Autodesk Inventor part; units mm, degrees
ref_plane "YZ Plane" through (0, 0, 0) normal (1, 0, 0) x (0, 1, 0)
ref_plane "XZ Plane" through (0, 0, 0) normal (0, 1, 0) x (-1, 0, 0)
ref_plane "XY Plane" through (0, 0, 0) normal (0, 0, 1) x (1, 0, 0)
sketch "Sketch1" plane through (0, 0, 0) normal (0, 0, 1) x (1, 0, 0)
  circle A0 centre (0, 0) radius 82.55
  circle A1 centre (0, 0) radius 101.6
  dimension "d0" = 203.2
  dimension "d1" = 19.05
extrude "Extrusion1" add sketch "Sketch1" along normal blind 4.7625
sketch "Sketch2" plane through (0, 0, 4.7625) normal (0, 0, 1) x (1, 0, 0)
  circle A0 centre (0, 0) radius 101.6
  line L0 (0, 0) -> (0, 92.075) construction
  circle A1 centre (0, 0) radius 92.075 construction
  circle A2 centre (0, 92.075) radius 3.175
  dimension "d4" = 9.525
  dimension "d5" = 6.35
extrude "Extrusion2" cut sketch "Sketch2" against normal through all contours A2
pattern_circular "Circular Pattern1" count 24 over 360 about axis through (0, 0, -10) along (0, 0, 1) of "Extrusion2"
properties part number "FlyWheelWeight" material "Aluminum-6061"
Can you work these out from the model? Positions are in its coordinate system, mm. Coordinates: 2 decimals unless noted, no trailing zeros. Write each loop counter-clockwise with the first axis right and the second up, starting at its lowest first coordinate (ties: lowest second). Pieces come first, ordered by that corner, then holes. Notation, with made-up numbers: M -24.75,-14.75 L 9.25,-14.75 A23 ccw 9.25,10.25 Z; hole C 12,-34.75 d8. An arc over 180 degrees is marked long. Answer as CSV lines item,"result".
Item 1: Imagine slicing it at A-A on y = 0. List the corners of the cut face in (x, z) for me, plus the area to 3 significant figures.
Geometry results:
outline,"M -101.6,0 L -95.25,0 L -95.25,4.76 L -101.6,4.76 Z; M -88.9,0 L -82.55,0 L -82.55,4.76 L -88.9,4.76 Z; M 82.55,0 L 88.9,0 L 88.9,4.76 L 82.55,4.76 Z; M 95.25,0 L 101.6,0 L 101.6,4.76 L 95.25,4.76 Z"
area,"121 mm2"
Item 2: Imagine slicing it at D-D on z = 2.2. State how many separate pieces and enclosed holes the cut face has, plus the area to 3 significant figures.
Geometry results:
separate pieces,"1"
enclosed holes,"25"
area,"10,300 mm2"
Item 3: Please list where these lines run through material, in increasing order: line 1 along Y through (x, z) = (0, 3.65); line 2 along X through (y, z) = (-68, 1.05); line 3 along Y through (x, z) = (65.5, 4.5).
Geometry results:
line 1,"y = -101.6 to -95.25, -88.9 to -82.55, 82.55 to 88.9, 95.25 to 101.6"
line 2,"x = -75.49 to -66.41, -63.8 to -46.8, 46.8 to 63.8, 66.41 to 75.49"
line 3,"y = -77.67 to -68.26, -61.96 to -50.24, 50.24 to 61.96, 68.26 to 77.67"
Item 4: I'm going to push flat-ended pins straight in: P1, Ø5.5, axis at x = 46.04, y = 79.74, coming from the -Z side; P2, Ø1.5, axis at x = -44.5, z = 1, coming from the -Y side. Where does each tip first touch, or does it pass through?
Geometry results:
P1,"passes through"
P2,"stops at y = -91.7"
Item 5: Imagine slicing it at C-C on y = 36. List the corners of the cut face in (x, z) for me.
Geometry results:
outline,"M -95.01,0 L -74.29,0 L -74.29,4.76 L -95.01,4.76 Z; M 74.29,0 L 95.01,0 L 95.01,4.76 L 74.29,4.76 Z"
Item 6: We'd pull the mould along Y, two halves only. Please class faces 1 (the cylindrical face through (76.567, -45.898, 2.415)), 2 (the cylindrical face through (-22.025, 99.184, 2.348)), 3 (the flat face through (-8, 83, 4.762)): +Y half, -Y half, draft (parallel to the pull), parting line (faces both ways), or undercut.
Geometry results:
face 1,"undercut"
face 2,"parting line"
face 3,"draft"
